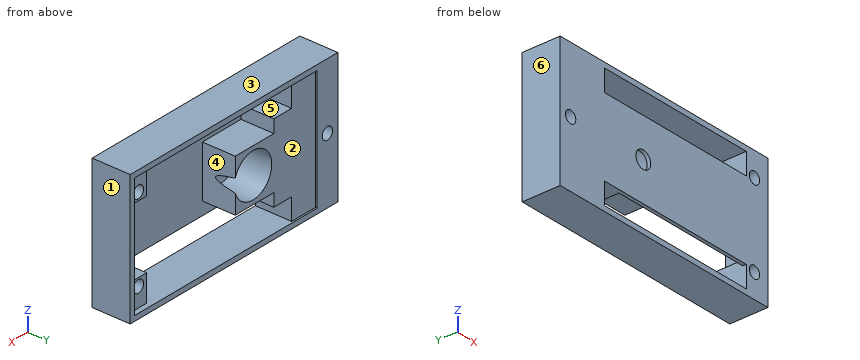
from build123d import *

# Parameters (mm, degrees)
SKETCH2_W               = 70
SKETCH2_H               = 38
SKETCH2_W_2             = 61.5
SKETCH2_H_2             = 35
SKETCH2_R               = 1.75
BOSS_EXTRUDE1_DEPTH     = 1
SKETCH2_3_W             = 70
SKETCH2_3_H             = 38
SKETCH2_3_W_2           = 61.5
SKETCH2_3_H_2           = 35
BOSS_EXTRUDE2_DEPTH     = 10
BOSS_EXTRUDE3_START     = 8.5
SKETCH2_4_R             = 1.75
BOSS_EXTRUDE3_DEPTH     = 8.5
CUT_EXTRUDE1_DEPTH      = 42.31585652
CUT_EXTRUDE1_DEPTH_BACK = 42.31585652
SKETCH3_R               = 1.75
BOSS_EXTRUDE4_DEPTH     = 10.5
SKETCH5_R               = 2.5
CUT_EXTRUDE2_DEPTH      = 1
SKETCH5_3_R             = 5.8
CUT_EXTRUDE3_DEPTH      = 42.060930335
CUT_EXTRUDE3_DRAFT      = -3


with BuildPart() as part:
    # Sketch2 → Boss-Extrude1 (new body)
    # profile 1 of 4: a face of its own
    with BuildSketch(Plane(origin=(0, 0, 0), x_dir=(1, 0, 0), z_dir=(0, 1, 0))):
        Rectangle(SKETCH2_W, SKETCH2_H)
        with Locations((2.75, 0)):
            Rectangle(SKETCH2_W_2, SKETCH2_H_2, mode=Mode.SUBTRACT)
    # profile 2 of 4: a face of its own
    with BuildSketch(Plane(origin=(0, 0, 0), x_dir=(1, 0, 0), z_dir=(0, 1, 0))):
        Polygon((27.75, 11.25), (-28, 11.25), (-28, -11.25), (27.75, -11.25), (27.75, -9.75), (33.5, -9.75), (33.5, 9.75), (27.75, 9.75), align=None)
    # profile 3 of 4: a face of its own
    with BuildSketch(Plane(origin=(0, 0, 0), x_dir=(1, 0, 0), z_dir=(0, 1, 0))):
        Polygon((33.5, 17.5), (27.75, 17.5), (27.75, 11.25), (27.75, 9.75), (33.5, 9.75), align=None)
        with Locations(Location((30.5, 12, 0), (0, 0, 270))):
            Circle(SKETCH2_R, mode=Mode.SUBTRACT)
    # profile 4 of 4: a face of its own
    with BuildSketch(Plane(origin=(0, 0, 0), x_dir=(1, 0, 0), z_dir=(0, 1, 0))):
        Polygon((27.75, -9.75), (27.75, -11.25), (27.75, -17.5), (33.5, -17.5), (33.5, -9.75), align=None)
        with Locations(Location((30.5, -12, 0), (0, 0, 270))):
            Circle(SKETCH2_R, mode=Mode.SUBTRACT)
    extrude(amount=-BOSS_EXTRUDE1_DEPTH)

    # Sketch2<3> → Boss-Extrude2 (add)
    with BuildSketch(Plane(origin=(0, 0, 0), x_dir=(1, 0, 0), z_dir=(0, 1, 0))):
        Rectangle(SKETCH2_3_W, SKETCH2_3_H)
        with Locations((2.75, 0)):
            Rectangle(SKETCH2_3_W_2, SKETCH2_3_H_2, mode=Mode.SUBTRACT)
    extrude(amount=BOSS_EXTRUDE2_DEPTH)

    # Sketch2<4> → Boss-Extrude3 (add)
    # profile 1 of 2: a face of its own
    with BuildSketch(Plane(origin=(0, 0, 0), x_dir=(1, 0, 0), z_dir=(0, 1, 0)).offset(BOSS_EXTRUDE3_START)):
        Polygon((33.5, 17.5), (27.75, 17.5), (27.75, 11.25), (27.75, 9.75), (33.5, 9.75), align=None)
        with Locations(Location((30.5, 12, 0), (0, 0, 270))):
            Circle(SKETCH2_4_R, mode=Mode.SUBTRACT)
    # profile 2 of 2: a face of its own
    with BuildSketch(Plane(origin=(0, 0, 0), x_dir=(1, 0, 0), z_dir=(0, 1, 0)).offset(BOSS_EXTRUDE3_START)):
        Polygon((27.75, -9.75), (27.75, -11.25), (27.75, -17.5), (33.5, -17.5), (33.5, -9.75), align=None)
        with Locations(Location((30.5, -12, 0), (0, 0, 270))):
            Circle(SKETCH2_4_R, mode=Mode.SUBTRACT)
    extrude(amount=-BOSS_EXTRUDE3_DEPTH)

    # Sketch3 → Cut-Extrude1 (cut, two sides: drawn at the far end of the back side and taken through both)
    with BuildSketch(Plane(origin=(0, 10, 0), x_dir=(1, 0, 0), z_dir=(0, 1, 0)).offset(-CUT_EXTRUDE1_DEPTH_BACK)):
        with Locations(Location((30.5, -12, 0), (0, 0, 270))):
            Circle(SKETCH3_R)
        with Locations(Location((30.5, 12, 0), (0, 0, 270))):
            Circle(SKETCH3_R)
        with Locations(Location((-31.5, 0, 0), (0, 0, 270))):
            Circle(SKETCH3_R)
    extrude(amount=CUT_EXTRUDE1_DEPTH + CUT_EXTRUDE1_DEPTH_BACK, mode=Mode.SUBTRACT)

    # Sketch4 → Boss-Extrude4 (add)
    with BuildSketch(Plane(origin=(0, -1, 0), x_dir=(1, 0, 0), z_dir=(0, 1, 0))):
        Polygon((-28, 17.5), (-20, 17.5), (-20, 11.25), (-14, 11.25), (-14, 7.5), (-1, 7.5), (-1, -7.5), (-14, -7.5), (-14, -11.25), (-20, -11.25), (-20, -17.5), (-28, -17.5), align=None)
    extrude(amount=BOSS_EXTRUDE4_DEPTH)

    # Sketch5 → Cut-Extrude2 (cut)
    with BuildSketch(Plane(origin=(0, 0, 0), x_dir=(1, 0, 0), z_dir=(0, 1, 0))):
        with Locations(Location((-7, 0, 0), (0, 0, 270))):
            Circle(SKETCH5_R)
    extrude(amount=-CUT_EXTRUDE2_DEPTH, mode=Mode.SUBTRACT)


with BuildPart() as cut_extrude3_tool:
    # Sketch5<3> → Cut-Extrude3 (with draft: the straight prism first)
    with BuildSketch(Plane(origin=(0, 0, 0), x_dir=(1, 0, 0), z_dir=(0, 1, 0))):
        with Locations((-7, 0)):
            Circle(SKETCH5_3_R)
    extrude(amount=CUT_EXTRUDE3_DEPTH)
    # Cut-Extrude3: the draft: its side faces are tilted about the plane it starts from
    cut_extrude3_sides = [cut_extrude3_tool.faces().sort_by_distance(p)[0] for p in [
        (-12.8, 21.030465168, 0),
    ]]
    draft(cut_extrude3_sides, Plane(origin=(0, 0, 0), x_dir=(1, 0, 0), z_dir=(0, 1, 0)), CUT_EXTRUDE3_DRAFT)


with BuildPart() as part_1:
    add(part.part)

    # Cut-Extrude3: cut by cut_extrude3_tool
    add(cut_extrude3_tool.part, mode=Mode.SUBTRACT)


solid = part_1.part
The model under review builds one solid part; all positions refer to its coordinate system, in mm. Face numbers are marked on the shaded views. A direction names the side the tool comes from. Coordinates: 2 decimals unless noted, no trailing zeros. Order: outer loops, then holes, each group sorted by start corner. A loop starts at its lowest first (then second) coordinate and runs counter-clockwise, first axis right, second up. Notation, with made-up numbers: (75.5, 33.25) -> (129.5, 33.25) arc R26 ccw to (129.5, 48.25) -> close; hole circle Ø1 at (45.5, -37). An arc over 180 degrees is marked (long way). Answer in a Markdown table with one row per item.
(1) The part is to be moulded in two halves that separate along Z. For the marked faces 1, 2 and 3, say which applies: +Z half, -Z half, draft (parallel to the pull), parting line (faces both ways), or undercut.
Answers:
| item | result |
|---|---|
| face 1 | draft |
| face 2 | undercut |
| face 3 | +Z half |
(2) Consider section B-B (x = 30.5). Write out the cut boundary in (y, z), plus the area to 3 significant figures.
Answers:
| item | result |
|---|---|
| outline | (-1, -19) -> (10, -19) -> (10, -17.5) -> (8.5, -17.5) -> (8.5, -13.75) -> (-1, -13.75) -> close; (-1, -10.25) -> (8.5, -10.25) -> (8.5, -9.75) -> (0, -9.75) -> (0, 9.75) -> (8.5, 9.75) -> (8.5, 10.25) -> (-1, 10.25) -> close; (-1, 13.75) -> (8.5, 13.75) -> (8.5, 17.5) -> (10, 17.5) -> (10, 19) -> (-1, 19) -> close |
| area | 133 mm² |
(3) Consider section D-D (y = 7.25). Write out the cut boundary in (x, z).
Answers:
| item | result |
|---|---|
| outline | (-35, -19) -> (35, -19) -> (35, 19) -> (-35, 19) -> close; hole circle Ø3.5 at (-31.5, 0); hole (-20, -17.5) -> (27.75, -17.5) -> (27.75, -9.75) -> (33.5, -9.75) -> (33.5, 9.75) -> (27.75, 9.75) -> (27.75, 17.5) -> (-20, 17.5) -> (-20, 11.25) -> (-14, 11.25) -> (-14, 7.5) -> (-1, 7.5) -> (-1, 1.48) arc R6.18 ccw (long way) to (-1, -1.48) -> (-1, -7.5) -> (-14, -7.5) -> (-14, -11.25) -> (-20, -11.25) -> close; hole circle Ø3.5 at (30.5, -12); hole circle Ø3.5 at (30.5, 12) |
(4) Wall thickness on line 1 along X through (y, z) = (4.25, 12); line 2 along X through (y, z) = (-0.5, 0); line 3 along Z through (x, y) = (24.5, 2): over which ranges is each line inside the solid? List them lowest first.
Answers:
| item | result |
|---|---|
| line 1 | -35 to -20, 27.75 to 28.75, 32.25 to 35 |
| line 2 | -35 to -33.25, -29.75 to -9.5, -4.5 to 35 |
| line 3 | -19 to -17.5, 17.5 to 19 |
(5) Consider section C-C (x = -7). Write out the cut boundary in (y, z), plus the area to 3 significant figures.
Answers:
| item | result |
|---|---|
| outline | (-1, -19) -> (10, -19) -> (10, -17.5) -> (-1, -17.5) -> close; (-1, -11.25) -> (0, -11.25) -> (0, -7.5) -> (9.5, -7.5) -> (9.5, -6.3) -> (0, -5.8) -> (0, -2.5) -> (-1, -2.5) -> close; (-1, 2.5) -> (0, 2.5) -> (0, 5.8) -> (9.5, 6.3) -> (9.5, 7.5) -> (0, 7.5) -> (0, 11.25) -> (-1, 11.25) -> close; (-1, 17.5) -> (10, 17.5) -> (10, 19) -> (-1, 19) -> close |
| area | 78.1 mm² |
(6) Machinability: for the marked faces 4, 5 and 6, which of the approach directions +Z, -Z, +X, -X, +Y, -Y give a long, thin tool a straight path to every point of the face, cutting with its end or side? Answer none if there is none.
Answers:
| item | result |
|---|---|
| face 4 | +Y |
| face 5 | +Y, -Y |
| face 6 | +Z, -Z, -X, +Y, -Y |
(7) Consider section A-A (z = -12). Write out the cut boundary in (x, y), plus the area to 3 significant figures.
Answers:
| item | result |
|---|---|
| outline | (-35, -1) -> (-20, -1) -> (-20, 9.5) -> (-28, 9.5) -> (-28, 10) -> (-35, 10) -> close; (27.75, -1) -> (28.75, -1) -> (28.75, 8.5) -> (27.75, 8.5) -> close; (32.25, -1) -> (35, -1) -> (35, 10) -> (33.5, 10) -> (33.5, 8.5) -> (32.25, 8.5) -> close |
| area | 199 mm² |
(8) Insertion check: pin 1 (1 mm diameter, centred on x = -9, z = -1.5, fed in from +Y); pin 2 (8 mm diameter, centred on x = -1.5, z = 5, fed in from +Y); pin 3 (6.5 mm diameter, centred on x = 29.5, z = 12.5, fed in from +Y). Each pin has a flat end and moves straight along its axis. Give the tip position at first contact, or say it passes through.
Answers:
| item | result |
|---|---|
| pin 1 | y = 0 |
| pin 2 | y = 9.5 |
| pin 3 | y = 8.5 |
